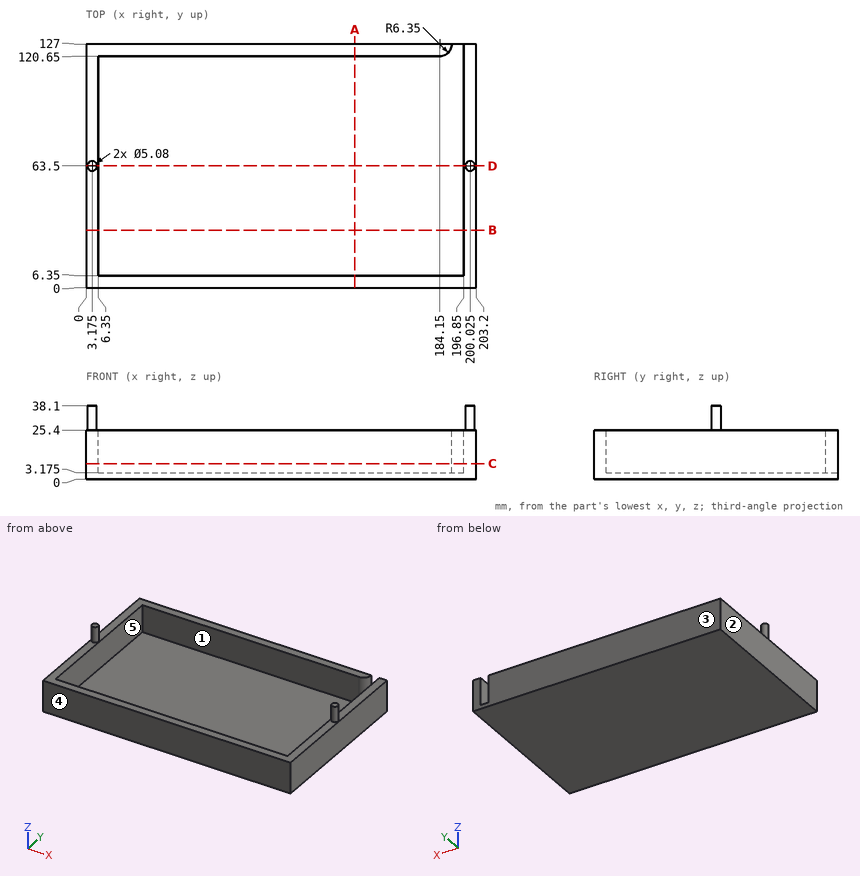
Input: dimensioned drawing with shaded views. Units: mm. Origin: part minimum x, y, z. A direction names the side the tool comes from. Give positions to 0.01 mm unless a question says otherwise; leave off trailing zeros. Order: outer loops, then holes, each group sorted by start corner. A loop starts at its lowest first (then second) coordinate and runs counter-clockwise, first axis right, second up. Notation, with made-up numbers: (7.25, 42.25) -> (57.25, 42.25) arc R13 ccw to (57.25, 59.25) -> close; hole circle Ø4 at (11, 47). An arc over 180 degrees is marked (long way). Answer as a JSON object with one key per item and string values.
Q1. Section D-D (y = 63.5). Output: boundary loops of the cut face in (x, z) (3 decimals), plus the area to 3 significant figures.
Entries:
{"outline": "(0, 0) -> (203.2, 0) -> (203.2, 25.4) -> (202.565, 25.4) -> (202.565, 38.1) -> (197.485, 38.1) -> (197.485, 25.4) -> (196.85, 25.4) -> (196.85, 3.175) -> (6.35, 3.175) -> (6.35, 25.4) -> (5.715, 25.4) -> (5.715, 38.1) -> (0.635, 38.1) -> (0.635, 25.4) -> (0, 25.4) -> close", "area": "1,060 mm^2"}
Q2. Access query for the marked faces 4 and 5. Directions: +Z, -Z, +X, -X, +Y, -Y. A direction counts if a zero-diameter tool reaches every point of the face in a straight line with its end or side. Return the directions, or none.
Entries:
{"face 4": "+Z, -Z, +X, -X, -Y", "face 5": "+Z"}
Q3. Material intervals for probe 1 along Y at (x, z) = (181, 8); probe 2 along X at (y, z) = (73.5, 18.5); probe 3 along Z at (x, y) = (45.5, 24) (3 decimals), sorted ascending.
Entries:
{"probe 1": "y = 0 to 6.35, 120.65 to 127", "probe 2": "x = 0 to 6.35, 196.85 to 203.2", "probe 3": "z = 0 to 3.175"}
Q4. Section C-C (z = 8). Output: boundary loops of the cut face in (x, y), plus the area to 3 significant figures.
Entries:
{"outline": "(0, 0) -> (203.2, 0) -> (203.2, 127) -> (196.85, 127) -> (196.85, 6.35) -> (6.35, 6.35) -> (6.35, 120.65) -> (184.15, 120.65) arc R6.35 ccw to (190.5, 127) -> (0, 127) -> close", "area": "3,980 mm^2"}
Q5. Draft query along X for the marked faces 1, 2 and 3. Return one class per face: released by +X, released by -X, zero draft, split by the parting line, or undercut.
Entries:
{"face 1": "undercut", "face 2": "released by -X", "face 3": "zero draft"}
Q6. Section B-B (y = 30). Output: boundary loops of the cut face in (x, z) (3 decimals).
Entries:
{"outline": "(0, 0) -> (203.2, 0) -> (203.2, 25.4) -> (196.85, 25.4) -> (196.85, 3.175) -> (6.35, 3.175) -> (6.35, 25.4) -> (0, 25.4) -> close"}
Q7. First-contact query: pin 1 (11 mm diameter, centred on x = 66, z = 11.5, fed in from -Y); pin 2 (8 mm diameter, centred on x = 161, y = 34, fed in from +Z) (3 decimals). Flat tips, straight axial feed; report the tip coordinate or a pass-through.
Entries:
{"pin 1": "stops at y = 0", "pin 2": "stops at z = 3.175"}
Q8. Section A-A (x = 140). Output: boundary loops of the cut face in (y, z) (3 decimals).
Entries:
{"outline": "(0, 0) -> (127, 0) -> (127, 25.4) -> (120.65, 25.4) -> (120.65, 3.175) -> (6.35, 3.175) -> (6.35, 25.4) -> (0, 25.4) -> close"}
